```python
from build123d import *
from OCP.BRepFilletAPI import BRepFilletAPI_MakeChamfer

# Parameters (mm, degrees)
SZKIC1_W                    = 31
SZKIC1_H                    = 43
DODANIE_WYCI_GNI_CIE1_DEPTH = 12
DODANIE_WYCI_GNI_CIE3_DEPTH = 5
SZKIC4_W                    = 5
SZKIC4_H                    = 43
WYTNIJ_WYCI_GNI_CIE1_DEPTH  = 5
DODANIE_WYCI_GNI_CIE4_DEPTH = 3.5
SZKIC6_W                    = 21
SZKIC6_H                    = 6
WYTNIJ_WYCI_GNI_CIE2_DEPTH  = 4
SFAZOWANIE1_SIZE2           = 3.356398525
SFAZOWANIE1_SIZE            = 4
SFAZOWANIE2_SIZE            = 2.020725942
SFAZOWANIE2_SIZE_2          = 3.5
ZAOKR_GLENIE2_R             = 2
SZKIC7_W                    = 2
SZKIC7_H                    = 1.5
DODANIE_WYCI_GNI_CIE5_DEPTH = 3
SFAZOWANIE3_SIZE            = 3
SFAZOWANIE3_SIZE_2          = 0.803847577


with BuildPart() as part:
    # Szkic1 → Dodanie-wyciągnięcie1 (new body)
    with BuildSketch(Plane(origin=(0, 0, 0), x_dir=(1, 0, 0), z_dir=(0, 1, 0))):
        Rectangle(SZKIC1_W, SZKIC1_H)
    extrude(amount=DODANIE_WYCI_GNI_CIE1_DEPTH)


with BuildPart() as body_2:
    # Szkic3 → Dodanie-wyciągnięcie3 (new body)
    with BuildSketch(Plane.XZ):
        with BuildLine():
            Line((-10.212337084, 28.112329696), (-14.125358878, 33.459474506))
            ThreePointArc((-14.125358878, 33.459474506), (-14.461615087, 35.767305941), (-12.741502742, 37.342224254))
            ThreePointArc((-12.741502742, 37.342224254), (-8.998415843, 41.011293853), (-10.279093338, 46.09387552))
            Line((-10.279093338, 46.09387552), (-15.166024728, 51.154438355))
            ThreePointArc((-15.166024728, 51.154438355), (-15.686793901, 52.037661779), (-15.750705614, 53.06098941))
            ThreePointArc((-15.750705614, 53.06098941), (-13.686472686, 56.384695233), (-10.429010158, 58.55195522))
            ThreePointArc((-10.429010158, 58.55195522), (-9.157993267, 58.652708308), (-8.044536022, 58.031541594))
            Line((-8.044536022, 58.031541594), (-4.224518095, 54.075788657))
            ThreePointArc((-4.224518095, 54.075788657), (0.407878305, 52.061536199), (5.107784388, 53.912803922))
            Line((5.107784388, 53.912803922), (9.063616274, 57.732769227))
            ThreePointArc((9.063616274, 57.732769227), (9.946850008, 58.253523329), (10.970179942, 58.317417838))
            ThreePointArc((10.970179942, 58.317417838), (12.642937927, 57.562348173), (14.103566869, 56.451126968))
            ThreePointArc((14.103566869, 56.451126968), (15.47806196, 54.856926305), (16.461051962, 52.995624834))
            ThreePointArc((16.461051962, 52.995624834), (16.56178137, 51.724613884), (15.94059861, 50.611174515))
            Line((15.94059861, 50.611174515), (10.879953282, 45.72434942))
            ThreePointArc((10.879953282, 45.72434942), (9.272518926, 41.94367997), (10.871160741, 38.159284239))
            ThreePointArc((10.871160741, 38.159284239), (11.521401414, 37.62253212), (12.248997344, 37.19648056))
            ThreePointArc((12.248997344, 37.19648056), (13.149955836, 36.868062858), (13.971590322, 36.373592268))
            ThreePointArc((13.971590322, 36.373592268), (14.805880692, 34.730389937), (14.282706099, 32.963346456))
            ThreePointArc((14.282706099, 32.963346456), (9.465690514, 26.653949977), (5.828617709, 19.59818464))
            ThreePointArc((5.828617709, 19.59818464), (4.786614899, 15.065901025), (4.553521224, 10.421223215))
            Line((4.553521224, 10.421223215), (7.14350853, -58.109023822))
            ThreePointArc((7.14350853, -58.109023822), (7.019012284, -59.657823394), (6.535877134, -61.134596855))
            Line((6.535877134, -61.134596855), (1.314918151, -72.39460248))
            ThreePointArc((1.314918151, -72.39460248), (-1.069105556, -73.746830857), (-3.119902204, -71.928500927))
            Line((-3.119902204, -71.928500927), (-5.8858069, -59.829088544))
            ThreePointArc((-5.8858069, -59.829088544), (-6.014905284, -59.054960819), (-6.051200692, -58.27098201))
            Line((-6.051200692, -58.27098201), (-5.119340887, 12.172423843))
            ThreePointArc((-5.119340887, 12.172423843), (-6.369476529, 20.556580537), (-10.212337084, 28.112329696))
        make_face()
    extrude(amount=-DODANIE_WYCI_GNI_CIE3_DEPTH)


with BuildPart() as part_1:
    add(part.part)

    # Połącz1: cut body 2
    add(body_2.part, mode=Mode.SUBTRACT)

    # Szkic4 → Wytnij-wyciągnięcie1 (cut)
    with BuildSketch(Plane.XZ):
        with Locations((13, 0)):
            Rectangle(SZKIC4_W, SZKIC4_H)
        with Locations((-13, 0)):
            Rectangle(SZKIC4_W, SZKIC4_H)
    extrude(amount=-WYTNIJ_WYCI_GNI_CIE1_DEPTH, mode=Mode.SUBTRACT)

    # Szkic5 → Dodanie-wyciągnięcie4 (add)
    with BuildSketch(Plane(origin=(0, 12, 0), x_dir=(1, 0, 0), z_dir=(0, 1, 0))):
        Polygon((10.5, 19.5), (10.5, 21.5), (15.5, 21.5), (15.5, -21.5), (11.5, -21.5), (11.5, -19.5), (13.5, -19.5), (13.5, 19.5), align=None)
        Polygon((-15.5, 21.5), (-15.5, -21.5), (-11.5, -21.5), (-11.5, -19.5), (-13.5, -19.5), (-13.5, 19.5), (-10.5, 19.5), (-10.5, 21.5), align=None)
    extrude(amount=DODANIE_WYCI_GNI_CIE4_DEPTH)

    # Szkic6 → Wytnij-wyciągnięcie2 (cut)
    with BuildSketch(Plane(origin=(0, 12, 0), x_dir=(1, 0, 0), z_dir=(0, 1, 0))):
        with Locations((0, 18.5)):
            Rectangle(SZKIC6_W, SZKIC6_H)
    extrude(amount=-WYTNIJ_WYCI_GNI_CIE2_DEPTH, mode=Mode.SUBTRACT)

    # Sfazowanie1
    sfazowanie1_edges = [part_1.edges().sort_by_distance(p)[0] for p in [
        (0, 8, -15.5),
    ]]
    sfazowanie1_side = [part_1.faces().sort_by_distance(p)[0] for p in [
        (0, 8.06712797, -15.5),
    ]]
    chamfer(sfazowanie1_edges, length=SFAZOWANIE1_SIZE - 0.0001, length2=SFAZOWANIE1_SIZE2 - 0.0001, reference=sfazowanie1_side[0])  # a hair under: the kernel refuses the full size

    # Sfazowanie2
    sfazowanie2_edges_1 = [part_1.edges().sort_by_distance(p)[0] for p in [
        (12, 12, -19.5),
    ]]
    sfazowanie2_side_1 = [part_1.faces().sort_by_distance(p)[0] for p in [
        (12, 12, -19.459585481),
    ]]
    sfazowanie2_edges_2 = [part_1.edges().sort_by_distance(p)[0] for p in [
        (-12, 12, -19.5),
    ]]
    sfazowanie2_side_2 = [part_1.faces().sort_by_distance(p)[0] for p in [
        (-12, 12, -19.459585481),
    ]]
    sfazowanie2 = BRepFilletAPI_MakeChamfer(part_1.part.solid().wrapped)
    for e in sfazowanie2_edges_1:
        sfazowanie2.Add(SFAZOWANIE2_SIZE - 0.0001, SFAZOWANIE2_SIZE_2 - 0.0001, e.wrapped, sfazowanie2_side_1[0].wrapped)
    for e in sfazowanie2_edges_2:
        sfazowanie2.Add(SFAZOWANIE2_SIZE - 0.0001, SFAZOWANIE2_SIZE_2 - 0.0001, e.wrapped, sfazowanie2_side_2[0].wrapped)
    add(Compound.cast(sfazowanie2.Shape()), mode=Mode.REPLACE)  # a hair under: the kernel refuses the full size

    # Zaokrąglenie2
    zaokr_glenie2_edges = [part_1.edges().sort_by_distance(p)[0] for p in [
        (-6.690658064, 2.5, 21.5),
        (6.65719404, 2.5, 21.5),
    ]]
    fillet(zaokr_glenie2_edges, radius=ZAOKR_GLENIE2_R)

    # Szkic7 → Dodanie-wyciągnięcie5 (add)
    with BuildSketch(Plane(origin=(0, 0, 19.5), x_dir=(-1, 0, 0), z_dir=(0, 0, -1))):
        with Locations((12.5, 14.75)):
            Rectangle(SZKIC7_W, SZKIC7_H)
        with Locations((-12.5, 14.75)):
            Rectangle(SZKIC7_W, SZKIC7_H)
    extrude(amount=DODANIE_WYCI_GNI_CIE5_DEPTH)

    # Sfazowanie3
    sfazowanie3_edges_1 = [part_1.edges().sort_by_distance(p)[0] for p in [
        (-12.5, 14, 16.5),
    ]]
    sfazowanie3_side_1 = [part_1.faces().sort_by_distance(p)[0] for p in [
        (-12.5, 14, 16.516076952),
    ]]
    sfazowanie3_edges_2 = [part_1.edges().sort_by_distance(p)[0] for p in [
        (12.5, 14, 16.5),
    ]]
    sfazowanie3_side_2 = [part_1.faces().sort_by_distance(p)[0] for p in [
        (12.5, 14, 16.516076952),
    ]]
    sfazowanie3 = BRepFilletAPI_MakeChamfer(part_1.part.solid().wrapped)
    for e in sfazowanie3_edges_1:
        sfazowanie3.Add(SFAZOWANIE3_SIZE - 0.0001, SFAZOWANIE3_SIZE_2 - 0.0001, e.wrapped, sfazowanie3_side_1[0].wrapped)
    for e in sfazowanie3_edges_2:
        sfazowanie3.Add(SFAZOWANIE3_SIZE - 0.0001, SFAZOWANIE3_SIZE_2 - 0.0001, e.wrapped, sfazowanie3_side_2[0].wrapped)
    add(Compound.cast(sfazowanie3.Shape()), mode=Mode.REPLACE)  # a hair under: the kernel refuses the full size


solid = part_1.part
```
Geometry: final body of the model. Coordinates: model frame, mm. A direction names the side the tool comes from. Round coordinates to 2 decimals unless told otherwise and drop trailing zeros. Loops run counter-clockwise (first coordinate to the right, second up) from the corner with the lowest first, then second, coordinate; pieces in that order, holes last.
Item 1: Section D-D, the plane y = 11. Output: boundary loops of the cut face in (x, z).
Checked values:
outline: (-15.5, -21.5) - (-10.5, -21.5) - (-10.5, -16.34) - (10.5, -16.34) - (10.5, -21.5) - (15.5, -21.5) - (15.5, 21.5) - (-15.5, 21.5) - close
Item 2: Line query: L1, parallel to X at y = 13.5, z = 6.5; L2, parallel to X at y = 10.75, z = -18; L3, parallel to Y at x = -6, z = -3. Output: solid intervals per line, ascending.
Checked values:
L1: x = -15.5 to -13.5, 13.5 to 15.5
L2: x = -15.5 to -10.5, 10.5 to 15.5
L3: y = 0 to 12
Item 3: Contact query for flat-ended pins moving along their axis: P1, Ø17.5, axis at x = 1, z = 9.5, coming from the -Y side; P2, Ø2.5, axis at x = -12.5, z = 7.5, coming from the -Y side; P3, Ø4, axis at y = 1.5, z = -3.5, coming from the +X side; P4, Ø2, axis at x = 9.5, z = -1, coming from the +Y side. Output: stop coordinate, or through.
Checked values:
P1: stops at y = 0
P2: stops at y = 5
P3: stops at x = 10.5
P4: stops at y = 12
Item 4: Reachability of faces 4 (the flat face through (-12.02, 13.77, -18.5)), 5 (the flat face through (0, 8, -20)), 6 (the flat face through (12, 13, 19.5)), 7 (the cylindrical face through (-6.956, 2.465, 21.114)) from +Z, -Z, +X, -X, +Y, -Y: full face, straight path, thin tool, end or side. Return the list, or none.
Checked values:
face 4: +Y
face 5: -Z, +Y
face 6: none
face 7: +Z, -Y
Item 5: Section A-A, the plane y = 1.75. Output: boundary loops of the cut face in (x, z), plus the area to 3 significant figures.
Checked values:
outline: (-10.5, -21.5) - (-5.56, -21.5) - (-5.12, 12.17) arc R26.4 ccw to (-6.22, 20.07) arc R2 ccw to (-8.14, 21.5) - (-10.5, 21.5) - close; (4.55, 10.42) - (5.76, -21.5) - (10.5, -21.5) - (10.5, 21.5) - (7.96, 21.5) arc R2 ccw to (6.12, 20.29) arc R45.13 ccw to (5.83, 19.6) arc R26.48 ccw to start
area: 448 mm2
Item 6: Section C-C, the plane z = 14. Output: boundary loops of the cut face in (x, y), plus the area to 3 significant figures.
Checked values:
outline: (-15.5, 5) - (-10.5, 5) - (-10.5, 0) - (-5.16, 0) - (-5.16, 5) - (4.66, 5) - (4.66, 0) - (10.5, 0) - (10.5, 5) - (15.5, 5) - (15.5, 15.5) - (13.5, 15.5) - (13.5, 12) - (-13.5, 12) - (-13.5, 15.5) - (-15.5, 15.5) - close
area: 287 mm2
Item 7: Mould query, pull axis X, two halves, no side actions, for faces 1 (the flat face through (-0.2, 7.6, -21.5)), 2 (the flat face through (10.5, 2, 0)), 3 (the flat face through (0, 12, 2)). Classes: released by +X, released by -X, zero draft, split by the parting line, or undercut.
Checked values:
face 1: zero draft
face 2: released by +X
face 3: undercut
